Model file for the job. Use its own axes, mm. Give positions to 0.01 mm unless a question says otherwise; leave off trailing zeros. Loops run counter-clockwise (first coordinate to the right, second up) from the corner with the lowest first, then second, coordinate; pieces in that order, holes last. Notation, with made-up numbers: M -34.5,-37.75 L 14.5,-37.75 A11 cw 14.5,-31.75 Z; hole C 25.25,36 d2. An arc over 180 degrees is marked long. Answer in a Markdown table with one row per item.
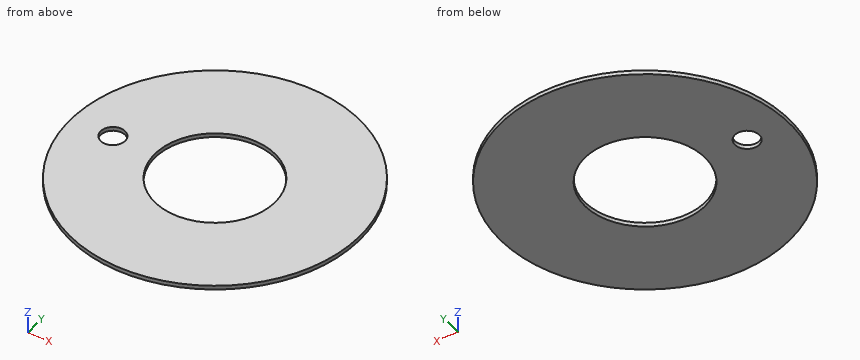
```python
from build123d import *

# Parameters (mm, degrees)
ESBO_O2_R                = 35.5
RESSALTO_EXTRUS_O1_DEPTH = 1
ESBO_O3_R                = 14.75
CORTE_EXTRUS_O1_DEPTH    = 1
ESBO_O7_R                = 3
CORTE_EXTRUS_O3_DEPTH    = 1


with BuildPart() as part:
    # Esboço2 → Ressalto-extrusão1 (new body)
    with BuildSketch(Plane.XY):
        Circle(ESBO_O2_R)
    extrude(amount=RESSALTO_EXTRUS_O1_DEPTH)

    # Esboço3 → Corte-extrusão1 (cut)
    with BuildSketch(Plane.XY.offset(1)):
        Circle(ESBO_O3_R)
    extrude(amount=-CORTE_EXTRUS_O1_DEPTH, mode=Mode.SUBTRACT)

    # Esboço7 → Corte-extrusão3 (cut)
    with BuildSketch(Plane.XY.offset(1)):
        with Locations((-25.203573784, 0)):
            Circle(ESBO_O7_R)
    extrude(amount=-CORTE_EXTRUS_O3_DEPTH, mode=Mode.SUBTRACT)


solid = part.part
```
Q1. Saw through at D-D (x = 8). Give the cut face in (y, z).
Reported:
| item | result |
|---|---|
| outline | M -34.59,0 L -12.39,0 L -12.39,1 L -34.59,1 Z; M 12.39,0 L 34.59,0 L 34.59,1 L 12.39,1 Z |
Q2. Saw through at C-C (z = 0.55). Give the cut face in (x, y).
Reported:
| item | result |
|---|---|
| outline | C 0,0 d71; hole C -25.2,0 d6; hole C 0,0 d29.5 |
Q3. Saw through at A-A (x = 0). Give the cut face in (y, z), and give its area (3 significant figures).
Reported:
| item | result |
|---|---|
| outline | M -35.5,0 L -14.75,0 L -14.75,1 L -35.5,1 Z; M 14.75,0 L 35.5,0 L 35.5,1 L 14.75,1 Z |
| area | 41.5 mm² |
Q4. Saw through at B-B (y = 0). Give the cut face in (x, z), and give its area (3 significant figures).
Reported:
| item | result |
|---|---|
| outline | M -35.5,0 L -28.2,0 L -28.2,1 L -35.5,1 Z; M -22.2,0 L -14.75,0 L -14.75,1 L -22.2,1 Z; M 14.75,0 L 35.5,0 L 35.5,1 L 14.75,1 Z |
| area | 35.5 mm² |
Q5. Probe probe 1 along Y at (x, z) = (0, 0.45); probe 2 along Y at (x, z) = (-5, 0.65); probe 3 along X at (y, z) = (-10.5, 0.6). List the from-to ranges inside material, lowest first.
Reported:
| item | result |
|---|---|
| probe 1 | -35.5 to -14.75, 14.75 to 35.5 |
| probe 2 | -35.15 to -13.88, 13.88 to 35.15 |
| probe 3 | -33.91 to -10.36, 10.36 to 33.91 |
